Work out the finished part from the listing and answer in its coordinate system (mm). Face numbers are marked on the shaded views. A direction names the side the tool comes from. Coordinates: 2 decimals unless noted, no trailing zeros. Order: outer loops, then holes, each group sorted by start corner. A loop starts at its lowest first (then second) coordinate and runs counter-clockwise, first axis right, second up. Notation, with made-up numbers: (16, 85) - (69, 85) arc R14 ccw to (69, 92) - close; hole circle Ø11 at (-4, -25.5). An arc over 180 degrees is marked (long way). Answer as a JSON object with one key per item and string values. Group by question number.
1) Section B-B (z = -8) is taken. Give the vertices of the cut face in (x, y), plus the area to 3 significant figures.
2) Find the intervals of material crossed by line 1 along Z through (x, y) = (1.75, -0.5); line 2 along Y through (x, z) = (0, -11.5); line 3 along X through (y, z) = (-0.75, -10.25), in increasing order.
3) Section A-A (y = 0) is taken. Give the vertices of the cut face in (x, z), plus the area to 3 significant figures.
4) The mould has two halves that part along Y. Classify the marked faces 1, 2 and 3: released by +Y, released by -Y, zero draft, split by the parting line, or undercut.
5) Each of these flat-tipped pins is pushed along its axis until it touches: P1, Ø3, axis at y = 1, z = -10, coming from the -X side; P2, Ø0.8, axis at y = 0.5, z = -1.5, coming from the -X side; P3, Ø4, axis at y = 2.5, z = -6.5, coming from the -X side; P4, Ø0.8, axis at x = -0.5, y = 0.5, coming from the +Z side. Where does it stop, or does it pass through?
6) A tool of negligible diameter and unlimited length cuts with its end or side. For the marked faces 4 and 5, from which of +Z, -Z, +X, -X, +Y, -Y can it reach the whole face along a straight path? Write none if from no direction.
from build123d import *

# Parameters (mm, degrees)
FOOTPRINT_DEPTH = 2.5
CHAMFER1_SIZE   = 0.5
FILLET1_R       = 1


with BuildPart() as part:
    # Sketch1 → Body (revolve)
    with BuildSketch(Plane(origin=(0, 0, 0), x_dir=(0, 0, -1), z_dir=(1, 0, 0)), mode=Mode.PRIVATE) as body_sk:
        Polygon((0, 0), (0, 3.5), (3, 3.5), (3, 1.5), (18, 1.5), (18, 0), align=None)
    revolve(body_sk.sketch.rotate(Axis((0, 0, 156.291575099), (0, 0, -1)), 90), axis=Axis((0, 0, 156.291575099), (0, 0, -1)))

    # Sketch2 → Footprint (cut)
    with BuildSketch(Plane.XY):
        Polygon((0, 1.5), (-1.299038106, 0.75), (-1.299038106, -0.75), (0, -1.5), (1.299038106, -0.75), (1.299038106, 0.75), align=None)
    extrude(amount=-FOOTPRINT_DEPTH, mode=Mode.SUBTRACT)

    # Chamfer1
    chamfer1_edges = [part.edges().sort_by_distance(p)[0] for p in [
        (-1.5, 0, -18),
    ]]
    chamfer(chamfer1_edges, length=CHAMFER1_SIZE)

    # Fillet1
    fillet1_edges = [part.edges().sort_by_distance(p)[0] for p in [
        (-3.5, 0, 0),
    ]]
    fillet(fillet1_edges, radius=FILLET1_R)


solid = part.part
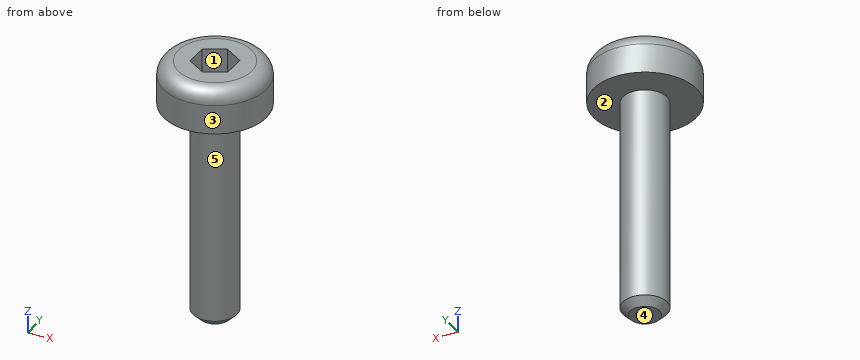
Report:
{
 "1": {"outline": "circle Ø3 at (0, 0)", "area": "7.07 mm²"},
 "2": {"line 1": "z = -3 to 0", "line 2": "y = -1.5 to 1.5", "line 3": "x = -1.3 to 1.3"},
 "3": {"outline": "(-3.5, -3) - (-1.5, -3) - (-1.5, -17.5) - (-1, -18) - (1, -18) - (1.5, -17.5) - (1.5, -3) - (3.5, -3) - (3.5, -1) arc R1 ccw to (2.5, 0) - (1.3, 0) - (1.3, -2.5) - (-1.3, -2.5) - (-1.3, 0) - (-2.5, 0) arc R1 ccw to (-3.5, -1) - close", "area": "58.8 mm²"},
 "4": {"face 1": "undercut", "face 2": "zero draft", "face 3": "split by the parting line"},
 "5": {"P1": "stops at x = -1.5", "P2": "stops at x = -3.5", "P3": "stops at x = -1.41", "P4": "stops at z = -2.5"},
 "6": {"face 4": "-Z, +X, -X, +Y, -Y", "face 5": "-Z"}
}
